Source: CAD feature listing. Evaluate the final solid. Frame: model axes, mm. Give positions to 0.01 mm unless a question says otherwise; leave off trailing zeros. Write each loop counter-clockwise with the first axis right and the second up, starting at its lowest first coordinate (ties: lowest second). Pieces come first, ordered by that corner, then holes. Notation, with made-up numbers: (70, 67.25) -> (119, 67.25) arc R30 ccw to (119, 104.25) -> close; hole circle Ø1 at (-4.75, 81.25). An arc over 180 degrees is marked (long way). Use one line per item in the form item = value. Start each with the question number.
(1) Cut plane A-A, the plane z = 11.5. Output: boundary loops of the cut face in (x, y).
(2) Cut plane B-B, the plane x = 1.6. Count the separate pieces of the cut face and the enclosed holes in it, and give its area (3 significant figures).
(3) Material intervals for line 1 along Y through (x, z) = (2.8, -24); line 2 along Y through (x, z) = (2.35, -8); line 3 along Z through (x, y) = (2.05, -1), sorted ascending. Write a range as from..to.
(4) First-contact query: P1, Ø2.5, axis at y = -36.74, z = -7.01, coming from the +X side; P2, Ø1.5, axis at x = 1, y = -28, coming from the +Z side. Flat tips, straight axial feed; report the tip coordinate or a pass-through.
from build123d import *

# Parameters (mm, degrees)
SKETCH_R           = 40
SKETCH_R_2         = 28
PAD_DEPTH          = 3
SKETCH001_R        = 1.6
POCKET_DEPTH       = 5
POLARPATTERN_COUNT = 50
SKETCH002_R        = 1.6
SKETCH002_R_2      = 2.5
POCKET001_DEPTH    = 3.001


with BuildPart() as part:
    # Sketch → Pad (new body)
    with BuildSketch(Plane.YZ):
        Circle(SKETCH_R)
        Circle(SKETCH_R_2, mode=Mode.SUBTRACT)
    extrude(amount=PAD_DEPTH)

    # Sketch001 (on Face4 of Pad) → Pocket (cut)
    with BuildSketch(Plane.YZ.offset(3)):
        with Locations((0, 37.4)):
            Circle(SKETCH001_R)
    pocket = extrude(amount=-POCKET_DEPTH, mode=Mode.SUBTRACT)

    # PolarPattern: Pocket ×50 about axis
    polarpattern_axis = Axis((3, 0, 0), (1, 0, 0))
    for i in range(1, POLARPATTERN_COUNT):
        add(pocket.rotate(polarpattern_axis, i * 360 / POLARPATTERN_COUNT), mode=Mode.SUBTRACT)

    # Sketch002 (on Face3 of PolarPattern) → Pocket001 (cut, through all)
    with BuildSketch(Plane.YZ.offset(3)):
        with Locations((1.997044, 31.742101)):
            Circle(SKETCH002_R)
        with Locations((31.804861, 0)):
            Circle(SKETCH002_R)
        with Locations((-31.804861, 0)):
            Circle(SKETCH002_R)
        with Locations((-1.997044, -31.742101)):
            Circle(SKETCH002_R)
        with Locations((22.817195, 21.948869)):
            Circle(SKETCH002_R_2)
    extrude(amount=-POCKET001_DEPTH, mode=Mode.SUBTRACT)


solid = part.part
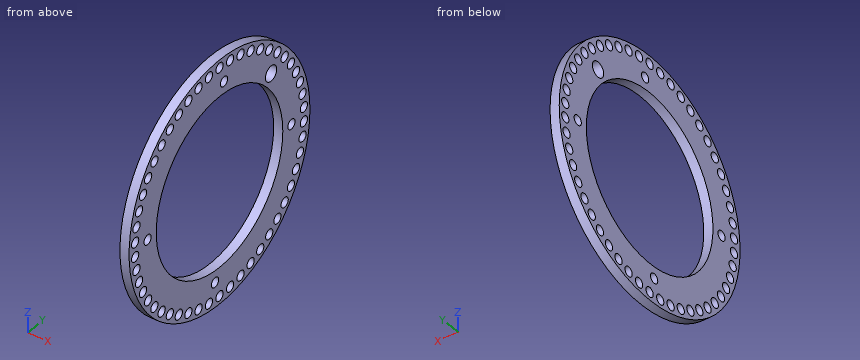
Geometry says:
q1.outline = (0, -38.31) -> (3, -38.31) -> (3, -37.17) -> (0, -37.17) -> close; (0, -33.97) -> (3, -33.97) -> (3, -25.53) -> (0, -25.53) -> close; (0, 25.53) -> (3, 25.53) -> (3, 33.97) -> (0, 33.97) -> close; (0, 37.17) -> (3, 37.17) -> (3, 38.31) -> (0, 38.31) -> close
q2.separate_pieces = 1
q2.enclosed_holes = 56
q2.area = 2,110 mm^2
q3.line_1 = -32..-30.41, -27.23..-14.42, 14.42..27.23, 30.41..32
q3.line_2 = -39.19..-37.99, -35.48..-26.83, 26.83..35.48, 37.99..39.19
q3.line_3 = -39.99..-38.65, -36.15..-32.99, -30.49..-27.98, 27.98..36.15, 38.65..39.99
q4.P1 = through
q4.P2 = 29.28
